Geometry check sheet. Reference: drawing and pictorial views, mm from the part's lowest x, y, z. A direction names the side the tool comes from. Round coordinates to 2 decimals unless told otherwise and drop trailing zeros. Write each loop counter-clockwise with the first axis right and the second up, starting at its lowest first coordinate (ties: lowest second). Pieces come first, ordered by that corner, then holes. Notation, with made-up numbers: (40, 17) - (53, 17) arc R18 ccw to (53, 26) - close; hole circle Ø7 at (21, 24.25). An arc over 180 degrees is marked (long way). Return JSON: item names as keys, results as strings.
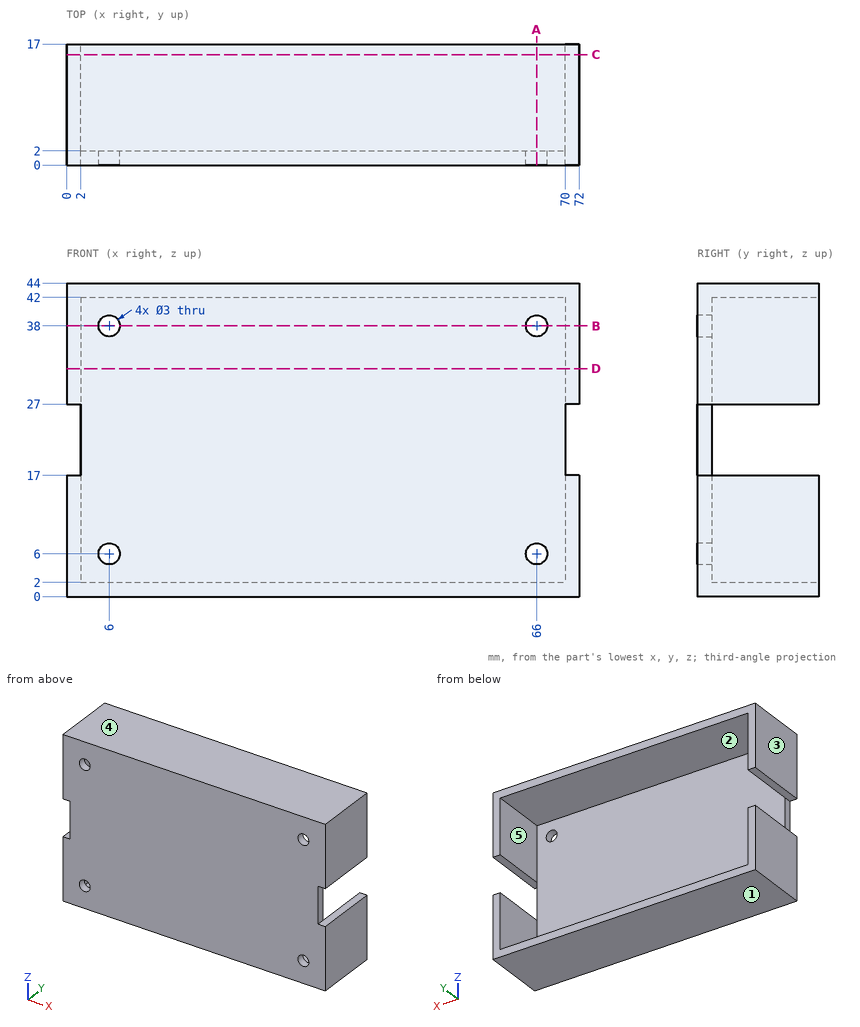
(1) Section check A-A, the plane x = 66. Enter the section's corners in (y, z), plus the area to 3 significant figures.
Response values:
{"outline": "(0, 0) - (17, 0) - (17, 2) - (2, 2) - (2, 4.5) - (0, 4.5) - close; (0, 7.5) - (2, 7.5) - (2, 36.5) - (0, 36.5) - close; (0, 39.5) - (2, 39.5) - (2, 42) - (17, 42) - (17, 44) - (0, 44) - close", "area": "136 mm^2"}
(2) Section check B-B, the plane z = 38. Enter the section's corners in (x, y), plus the area to 3 significant figures.
Response values:
{"outline": "(0, 0) - (4.5, 0) - (4.5, 2) - (2, 2) - (2, 17) - (0, 17) - close; (7.5, 0) - (64.5, 0) - (64.5, 2) - (7.5, 2) - close; (67.5, 0) - (72, 0) - (72, 17) - (70, 17) - (70, 2) - (67.5, 2) - close", "area": "192 mm^2"}
(3) Gauge pin test, flat ends, axial feed: pin 1 (4 mm diameter, centred on x = 66, z = 38, fed in from +Y); pin 2 (2.5 mm diameter, centred on x = 6, z = 38, fed in from +Y); pin 3 (0.6 mm diameter, centred on y = 0.5, z = 24, fed in from +X). Record the tip position at first contact, or that the pin passes through.
Response values:
{"pin 1": "stops at y = 2", "pin 2": "passes through", "pin 3": "stops at x = 70"}
(4) Section check C-C, the plane y = 15.5. Enter the section's corners in (x, z).
Response values:
{"outline": "(0, 0) - (72, 0) - (72, 17) - (70, 17) - (70, 2) - (2, 2) - (2, 17) - (0, 17) - close; (0, 27) - (2, 27) - (2, 42) - (70, 42) - (70, 27) - (72, 27) - (72, 44) - (0, 44) - close"}
(5) Material ranges on line 1 along Z through (x, y) = (66, 0.5); line 2 along X through (y, z) = (0.5, 6); line 3 along Z through (x, y) = (18.5, 14.5), recorded low to high. Write a range as [from, to].
Response values:
{"line 1": "z = [0, 4.5], [7.5, 36.5], [39.5, 44]", "line 2": "x = [0, 4.5], [7.5, 64.5], [67.5, 72]", "line 3": "z = [0, 2], [42, 44]"}
(6) Section check D-D, the plane z = 32. Enter the section's corners in (x, y), plus the area to 3 significant figures.
Response values:
{"outline": "(0, 0) - (72, 0) - (72, 17) - (70, 17) - (70, 2) - (2, 2) - (2, 17) - (0, 17) - close", "area": "204 mm^2"}
(7) Release check for a two-part mould opening along X. For the marked faces 3, 4 and 5 record: pulls with the +X half, pulls with the -X half, needs draft (parallel to the pull), parting line crosses it, or undercut.
Response values:
{"face 3": "pulls with the -X half", "face 4": "needs draft", "face 5": "undercut"}
(8) Access from +Z, -Z, +X, -X, +Y, -Y to the whole of each face (thin tool, end or side, straight path). Record for the marked faces 1 and 2.
Response values:
{"face 1": "-Z, +X, -X, +Y, -Y", "face 2": "+Y"}
